```python
from build123d import *

# Parameters (mm, degrees)
F1_DEPTH = 3.175
F2_SIZE  = 0.7874
F3_SIZE  = 0.7874
F4_SIZE  = 0.7874
F5_SIZE  = 0.7874
F6_SIZE  = 0.7874
F7_SIZE  = 0.7874


with BuildPart() as f1:
    # F0 (on Front) → F1 (new body)
    with BuildSketch(Plane.XZ):
        with BuildLine():
            Line((-30, 19.711864), (-30, -20.288136))
            Line((-30, -20.288136), (-5.722361, -20.288136))
            ThreePointArc((-5.722361, -20.288136), (-4.909056, -19.47483), (-4.09575, -20.288136))
            Line((-4.09575, -20.288136), (-2.802662, -25.288136))
            Line((-2.802662, -25.288136), (2.802662, -25.288136))
            Line((2.802662, -25.288136), (4.09575, -20.288136))
            ThreePointArc((4.09575, -20.288136), (4.909056, -19.47483), (5.722361, -20.288136))
            Line((5.722361, -20.288136), (30, -20.288136))
            Line((30, -20.288136), (30, -19.711864))
            Line((30, -19.711864), (30, 19.711864))
            Line((30, 19.711864), (5.60832, 19.711864))
            ThreePointArc((5.60832, 19.711864), (4.9022, 19.005744), (4.19608, 19.711864))
            Line((4.19608, 19.711864), (2.902992, 24.711864))
            Line((2.902992, 24.711864), (-2.902992, 24.711864))
            Line((-2.902992, 24.711864), (-4.19608, 19.711864))
            ThreePointArc((-4.19608, 19.711864), (-4.9022, 19.005744), (-5.60832, 19.711864))
            Line((-5.60832, 19.711864), (-30, 19.711864))
        make_face()
    extrude(amount=F1_DEPTH)

    # F2
    f2_edges = [f1.edges().sort_by_distance(p)[0] for p in [
        (-17.861181, 0, -20.288136),
        (17.861181, 0, -20.288136),
        (17.861181, -3.175, -20.288136),
        (-17.861181, -3.175, -20.288136),
    ]]
    chamfer(f2_edges, length=F2_SIZE)

    # F3
    f3_edges = [f1.edges().sort_by_distance(p)[0] for p in [
        (3.549536, 0, 22.211864),
        (4.9022, 0, 19.005744),
        (-3.549536, 0, 22.211864),
        (-4.9022, 0, 19.005744),
    ]]
    chamfer(f3_edges, length=F3_SIZE)

    # F4
    f4_edges = [f1.edges().sort_by_distance(p)[0] for p in [
        (4.9022, -3.175, 19.005744),
        (3.549536, -3.175, 22.211864),
        (-3.549536, -3.175, 22.211864),
        (-4.9022, -3.175, 19.005744),
    ]]
    chamfer(f4_edges, length=F4_SIZE)

    # F5
    f5_edges = [f1.edges().sort_by_distance(p)[0] for p in [
        (18.19786, -3.175, 19.711864),
        (-18.19786, -3.175, 19.711864),
        (18.19786, 0, 19.711864),
        (-18.19786, 0, 19.711864),
    ]]
    chamfer(f5_edges, length=F5_SIZE)

    # F6
    f6_edges = [f1.edges().sort_by_distance(p)[0] for p in [
        (3.449206, -3.175, -22.788136),
        (4.411136, -3.175, -19.645063),
        (-3.449206, -3.175, -22.788136),
        (-4.411136, -3.175, -19.645063),
    ]]
    chamfer(f6_edges, length=F6_SIZE)

    # F7
    f7_edges = [f1.edges().sort_by_distance(p)[0] for p in [
        (3.449206, 0, -22.788136),
        (4.411136, 0, -19.645063),
        (-3.449206, 0, -22.788136),
        (-4.411136, 0, -19.645063),
    ]]
    chamfer(f7_edges, length=F7_SIZE)


solid = f1.part
```
Design review of the part built by this model. Coordinates are the model's own, in mm. A direction names the side the tool comes from. Coordinates: 2 decimals unless noted, no trailing zeros. Order: outer loops, then holes, each group sorted by start corner. A loop starts at its lowest first (then second) coordinate and runs counter-clockwise, first axis right, second up.
1) Clearance check with flat-ended pins moving along their axes: pin 1 (1.8 mm diameter, centred on x = -20, y = -1.5, fed in from -Z); pin 2 (1 mm diameter, centred on x = -1, z = 0, fed in from +Y); pin 3 (1.3 mm diameter, centred on x = 16, y = -2, fed in from +Z). State where each tip first meets the part, or that it passes through.
2) Mouldability with a two-part tool opening along X and no side actions: class faces 3 (the conical face through (4.92, -0.57, 18.79)), 4 (the flat face through (-18, -2, -20.288)), 5 (the flat face through (-3.14, -0.4, 22.25)), 6 (the flat face through (3.559, -1.576, 22.177)) as +X half, -X half, draft (parallel to the pull), parting line (faces both ways), or undercut.
3) For faces 1 (the flat face through (18, -2, 19.712)), 2 (the flat face through (-3.06, -0.4, -22.75)), list the 3-axis set-ups (+Z, -Z, +X, -X, +Y, -Y) from which the entire face can be reached by the end or side of a thin tool; tool diameter is ignored.
4) Take a section at A-A, the plane y = -1.65. Give the boundary of the cut face in (x, z), and give its area (3 significant figures).
5) Wall thickness on line 1 along Z through (x, y) = (24, -1.25); line 2 along Z through (x, y) = (6.5, -2.55): over which ranges is each line inside the solid? List them lowest first.
6) Take a section at B-B, the plane z = 21.5. Give the boundary of the cut face in (x, y) (3 decimals).
7) Take a section at C-C, the plane x = 9. Give the boundary of the cut face in (y, z) (3 decimals).
Returned:
1. pin 1: stops at z = -20.29
1. pin 2: stops at y = 0
1. pin 3: stops at z = 19.71
2. face 3: undercut
2. face 4: draft
2. face 5: -X half
2. face 6: +X half
3. face 1: +Z, +X, +Y, -Y
3. face 2: -Z, -X, +Y
4. outline: (-30, -20.29) - (-5.72, -20.29) arc R0.81 cw to (-4.1, -20.29) - (-2.8, -25.29) - (2.8, -25.29) - (4.1, -20.29) arc R0.81 cw to (5.72, -20.29) - (30, -20.29) - (30, 19.71) - (5.61, 19.71) arc R0.71 cw to (4.2, 19.71) - (2.9, 24.71) - (-2.9, 24.71) - (-4.2, 19.71) arc R0.71 cw to (-5.61, 19.71) - (-30, 19.71) - close
4. area: 2,470 mm2
5. line 1: z = -20.29 to 19.71
5. line 2: z = -20.13 to 19.55
6. outline: (-3.734, -2.388) - (-2.92, -3.175) - (2.92, -3.175) - (3.734, -2.388) - (3.734, -0.787) - (2.92, 0) - (-2.92, 0) - (-3.734, -0.787) - close
7. outline: (-3.175, -19.501) - (-2.388, -20.288) - (-0.787, -20.288) - (0, -19.501) - (0, 18.924) - (-0.787, 19.712) - (-2.388, 19.712) - (-3.175, 18.924) - close
